For this review, take the finished solid that the model builds, in its own axes (mm). A direction names the side the tool comes from. Coordinates: 2 decimals unless noted, no trailing zeros. Write each loop counter-clockwise with the first axis right and the second up, starting at its lowest first coordinate (ties: lowest second). Pieces come first, ordered by that corner, then holes.
Autodesk Inventor part; units mm, degrees
ref_plane "YZ Plane" through (0, 0, 0) normal (1, 0, 0) x (0, 1, 0)
ref_plane "XZ Plane" through (0, 0, 0) normal (0, 1, 0) x (-1, 0, 0)
ref_plane "XY Plane" through (0, 0, 0) normal (0, 0, 1) x (1, 0, 0)
sketch "Sketch1" plane through (0, 0, 0) normal (0, 0, 1) x (1, 0, 0)
  circle A0 centre (0, 0) radius 37.5
  circle A1 centre (0, 0) radius 40.5
  point P0 (0, 0)
  dimension "d0" = 3
extrude "Extrusion1" add sketch "Sketch1" against normal blind 60
sketch "Sketch8" plane through (0, 0, 0) normal (0, 0, 1) x (1, 0, 0)
  line L0 (0, 0) -> (-46.6973, 0) construction
  line L1 (0, 0) -> (-40.4753, 1.4134) construction
  circle A0 centre (0, 0) radius 40.5
  line L2 (0, 0) -> (-40.4753, -1.4134) construction
  circle A1 centre (0, 0) radius 37.5
  line L3 (-37.4772, -1.3087) -> (-40.4753, -1.4134)
  line L4 (-37.4772, 1.3087) -> (-40.4753, 1.4134)
  dimension "d30" = 4
extrude "Extrusion9" cut sketch "Sketch8" against normal blind 40 contours L4 A1 L3 A0 picked at (-39.4973, -0.1454)
pattern_circular "Circular Pattern2" count 6 over 360 about axis through (0, 0, 0) along (0, 0, -1) of "Extrusion9"
sketch "Sketch9" plane through (21.4617, -34.3459, -40) normal (0, 0, 1) x (0.848, 0.5299, 0)
  circle A0 centre (0, 40.5) radius 37.5 construction
  circle A1 centre (0, 40.5) radius 40.5
  circle A2 centre (0, 40.5) radius 39.5
  point P0 (0, 40.5)
  dimension "d36" = 1
extrude "Extrusion10" cut sketch "Sketch9" along normal blind 12
sketch "Sketch10" plane through (0, 0, -60) normal (0, 0, -1) x (-1, 0, 0)
  line L0 (41, -41) -> (-41, -41)
  line L1 (-41, -41) -> (-41, 41)
  line L2 (-41, 41) -> (41, 41)
  line L3 (41, 41) -> (41, -41)
  line L4 (41, -41) -> (-41, 41) construction
  line L5 (-41, -41) -> (41, 41) construction
  circle A0 centre (0, 0) radius 37.5 construction
  circle A1 centre (0, 0) radius 35.5
  point P0 (0, 0)
  dimension "d39" = 82
  dimension "d40" = 82
  dimension "d41" = 2
extrude "Extrusion11" add sketch "Sketch10" along normal blind 4
sketch "Sketch11" plane through (0, 0, -60) normal (0, 0, 1) x (1, 0, 0)
  line L0 (-41, 41) -> (-41, -41) construction
  line L1 (-41, -41) -> (41, -41) construction
  line L2 (41, -41) -> (41, 41) construction
  line L3 (41, 41) -> (-41, 41) construction
  line L4 (-35, -35) -> (-35, 35) construction
  line L5 (-35, 35) -> (35, 35) construction
  line L6 (35, 35) -> (35, -35) construction
  line L7 (35, -35) -> (-35, -35) construction
  point P0 (0, 0)
  dimension "d44" = 6
hole "Hole1" at (-35, -35, -60) at (-35, 35, -60) at (35, 35, -60) at (35, -35, -60) direction (0, 0, -1) diameter 3 end through all
fillet "Fillet2" radius 2 1 edges at (-40.5, 0, -60)
sketch "Sketch7" plane through (0, 0, -5) normal (0, 0, -1) x (-1, 0, 0)
  circle A0 centre (0, 0) radius 40.5
  circle A1 centre (0, 0) radius 39.5
  point P0 (0, 0)
  dimension "d27" = 1
properties part number "Cup_Dispenser_Flip_Flop"
1) Clearance check with flat-ended pins moving along their axes: P1, Ø3, axis at y = 6, z = -44, coming from the -X side; P2, Ø5, axis at x = -35, y = -35, coming from the +Z side; P3, Ø1.5, axis at y = 23.5, z = -49, coming from the -X side; P4, Ø12, axis at x = -21.5, y = -11, coming from the -Z side. State where each tip first meets the part, or that it passes through.
2) The part is to be moulded in two halves that separate along Y. For faces 6 (the face through (-34.935, 20.489, -13.804)), 7 (the face through (-35.21, -20.01, -13.8)), 8 (the face through (7.696, 34.656, -61.972)), say which applies: pulls with the +Y half, pulls with the -Y half, needs draft (parallel to the pull), parting line crosses it, or undercut.
3) For L1, parallel to Y at x = 0, z = -63.2; L2, parallel to Z at x = 12, y = 35; L3, parallel to Y at x = 0, z = -15, list the stretches that pass through material, from the lowest coordinate up.
4) Consider section B-B (z = -31). Give the boundary of the cut face in (x, y).
5) Consider section C-C (z = -11.5). Give the boundary of the cut face in (x, y), then the cut area to 3 significant figures.
6) Consider section A-A (z = -45.5). Give the boundary of the cut face in (x, y).
7) Tool access review of faces 1 (the face through (33, 32, -60)), 2 (the face through (38, -1, -40)), 3 (the face through (34.072, 19.984, -34.084)), 4 (the face through (34.34, -19.52, -34.08)), 5 (the face through (-34.34, 19.52, -34.08)): name each direction out of +Z, -Z, +X, -X, +Y, -Y from which nothing blocks a thin tool from reaching the whole face with its end or side.
Results:
1. P1: stops at x = -40.25
1. P2: stops at z = -60
1. P3: stops at x = -33.51
1. P4: passes through
2. face 6: pulls with the +Y half
2. face 7: pulls with the -Y half
2. face 8: undercut
3. L1: y = -41 to -35.5, 35.5 to 41
3. L2: z = -64 to -60
3. L3: y = -40.5 to -37.5, 37.5 to 40.5
4. outline: (-39.48, -1.38) arc R39.5 ccw to (-20.93, -33.5) - (-19.87, -31.8) arc R37.5 cw to (-37.48, -1.31) - close; (-39.48, 1.38) - (-37.48, 1.31) arc R37.5 cw to (-19.87, 31.8) - (-20.93, 33.5) arc R39.5 ccw to start; (-18.54, -34.88) arc R39.5 ccw to (18.54, -34.88) - (17.61, -33.11) arc R37.5 cw to (-17.61, -33.11) - close; (-18.54, 34.88) - (-17.61, 33.11) arc R37.5 cw to (17.61, 33.11) - (18.54, 34.88) arc R39.5 ccw to start; (19.87, -31.8) - (20.93, -33.5) arc R39.5 ccw to (39.48, -1.38) - (37.48, -1.31) arc R37.5 cw to start; (19.87, 31.8) arc R37.5 cw to (37.48, 1.31) - (39.48, 1.38) arc R39.5 ccw to (20.93, 33.5) - close
5. outline: (-40.48, -1.41) arc R40.5 ccw to (-21.46, -34.35) - (-19.87, -31.8) arc R37.5 cw to (-37.48, -1.31) - close; (-40.48, 1.41) - (-37.48, 1.31) arc R37.5 cw to (-19.87, 31.8) - (-21.46, 34.35) arc R40.5 ccw to start; (-19.01, -35.76) arc R40.5 ccw to (19.01, -35.76) - (17.61, -33.11) arc R37.5 cw to (-17.61, -33.11) - close; (-19.01, 35.76) - (-17.61, 33.11) arc R37.5 cw to (17.61, 33.11) - (19.01, 35.76) arc R40.5 ccw to start; (19.87, -31.8) - (21.46, -34.35) arc R40.5 ccw to (40.48, -1.41) - (37.48, -1.31) arc R37.5 cw to start; (19.87, 31.8) arc R37.5 cw to (37.48, 1.31) - (40.48, 1.41) arc R40.5 ccw to (21.46, 34.35) - close
5. area: 686 mm2
6. outline: circle Ø81 at (0, 0); hole circle Ø75 at (0, 0)
7. face 1: +Z, +X, +Y
7. face 2: none
7. face 3: +X, +Y
7. face 4: +X, -Y
7. face 5: -X, +Y
